Work out the finished part from the listing and answer in its coordinate system (mm). Face numbers are marked on the shaded views. A direction names the side the tool comes from. Round coordinates to 2 decimals unless told otherwise and drop trailing zeros. Order: outer loops, then holes, each group sorted by start corner. A loop starts at its lowest first (then second) coordinate and runs counter-clockwise, first axis right, second up. Notation, with made-up numbers: M 6,59.25 L 32,59.25 A28 ccw 32,89.25 Z; hole C -30.5,-22 d8. An arc over 180 degrees is marked long. Return JSON: item names as keys, results as strings.
from build123d import *

# Parameters (mm, degrees)
F0_W        = 46
F0_H        = 72
F1_DEPTH    = 96
F2_W        = 42
F2_H        = 68
F3_DEPTH    = 92
F4_R        = 4
F5_DEPTH    = 3.2
F6_R        = 4
F7_DEPTH    = 3.2
F8_T1_DEPTH = 97.7168298797
F9_R        = 1
F10_R       = 27.7209608442
F11_DEPTH   = 2


# Not quite as in the source:
# - a fillet or chamfer that OpenCascade refuses, or shapes differently, is made with other operations: its cross-section is extruded or revolved along the edge and cut away or added


with BuildPart() as f1:
    # F0 (on Top) → F1 (new body)
    with BuildSketch(Plane.XY):
        Rectangle(F0_W, F0_H)
    extrude(amount=F1_DEPTH)

    # F2 (on face) → F3 (cut)
    with BuildSketch(Plane.XY.offset(96)):
        Rectangle(F2_W, F2_H)
    extrude(amount=-F3_DEPTH, mode=Mode.SUBTRACT)

    # F4 (on face) → F5 (join)
    with BuildSketch(Plane.XZ.offset(36)):
        with Locations((13, 82)):
            Circle(F4_R)
    extrude(amount=F5_DEPTH)

    # F6 (on face) → F7 (join)
    with BuildSketch(Plane(origin=(0, 36, 0), x_dir=(-1, 0, 0), z_dir=(0, 1, 0))):
        with Locations((-13, 82)):
            Circle(F6_R)
    extrude(amount=F7_DEPTH)

    # F8: chamfer of 5 on 1 edges, made by hand

    # F8_s2 → F8_t1 (cut)
    with BuildSketch(Plane.XZ.offset(-48.8584149398)):
        Polygon((-18, 96), (-23, 91), (-23, 96), align=None)
    extrude(amount=F8_T1_DEPTH, mode=Mode.SUBTRACT)

    # F9
    f9_edges = [f1.edges().sort_by_distance(p)[0] for p in [
        (-23, -36, 45.5),
        (23, -36, 48),
        (23, 36, 48),
        (-23, 36, 45.5),
        (23, 0, 0),
        (-23, 0, 0),
        (0, 36, 0),
        (0, -36, 0),
    ]]
    fillet(f9_edges, radius=F9_R)

    # F10 (on face) → F11 (join)
    with BuildSketch(Plane(origin=(-23, 0, 0), x_dir=(0, -1, 0), z_dir=(-1, 0, 0))):
        with Locations((0, 40.8182404935)):
            Circle(F10_R)
        with BuildLine():
            add(Edge.make_bspline(
                [(-17.8310812866, 24.7516158604), (-18.0416931886, 24.731624497), (-18.6386807496, 24.6684959969), (-19.2717295968, 24.3841029538), (-19.5649090195, 21.6870798509), (-16.5966593688, 21.0684697904), (-15.2211504824, 21.4407750456), (-14.5426337104, 21.7238514822)],
                knots=[0.4132110552, 0.4132110552, 0.4132110552, 0.4132110552, 0.4283251344, 0.4603190645, 0.510541782, 0.5666924956, 0.615415561, 0.615415561, 0.615415561, 0.615415561], degree=3))
            ThreePointArc((-17.8310812866, 24.7516158604), (-8.6054277875, 63.2242776163), (24.0017475812, 40.8182404935))
            ThreePointArc((24.0017475812, 40.8182404935), (22.6894322226, 32.9904980114), (18.8959899976, 26.0187320907))
            add(Edge.make_bspline(
                [(13.5544067846, 21.0101122713), (15.1773683066, 20.8286148298), (18.6415516168, 20.5611168513), (20.2513827461, 23.1969599021), (20.017563928, 26.727985113), (19.3356446095, 26.1886613097), (18.9151411243, 26.0259448267), (18.8959899976, 26.0187320907)],
                knots=[0.4868760993, 0.4868760993, 0.4868760993, 0.4868760993, 0.6035189288, 0.7106541171, 0.8124300784, 0.8685997483, 0.87123087, 0.87123087, 0.87123087, 0.87123087], degree=3))
            ThreePointArc((13.5544067846, 21.0101122713), (-0.6095113038, 16.8242332642), (-14.5426337104, 21.7238514822))
        make_face(mode=Mode.SUBTRACT)
        with BuildLine():
            add(Edge.make_bspline(
                [(-13.1672387943, 47.9557514191), (-13.6789435568, 47.7302779724), (-13.8554780387, 46.5012200329), (-11.906507855, 43.7928351191), (-10.8613262187, 42.8100774548), (-6.4416701192, 46.0388131445), (-5.8697363247, 48.1862573802), (-6.5496625571, 49.5720681387), (-8.0107671732, 47.5720952119), (-12.18493142, 48.3885873933), (-13.1672387943, 47.9557514191)],
                knots=[0, 0, 0, 0, 0.0951179589, 0.2427295185, 0.3289680533, 0.5102542132, 0.6320447089, 0.7083203168, 0.817404333, 1, 1, 1, 1], degree=3))
        make_face()
        with BuildLine():
            add(Edge.make_bspline(
                [(-1.5056377742, 51.0721281171), (-1.2655745051, 51.376089636), (-0.785072868, 51.9844876136), (0.4890633383, 51.9466317035), (1.1904519521, 51.3741917059), (1.5605587978, 51.0721281171)],
                knots=[0, 0, 0, 0, 0.3204609859, 0.6414226921, 1, 1, 1, 1], degree=3))
            Line((-1.5056377742, 51.0721281171), (-1.5056377742, 40.8182404935))
            Line((-1.5056377742, 40.8182404935), (-13.8206910342, 40.8182404935))
            add(Edge.make_bspline(
                [(-13.8206910342, 40.8182404935), (-14.3163583008, 40.7406958322), (-15.3248298347, 40.5829255117), (-16.0298313022, 38.9853309187), (-15.2661185632, 37.3287424191), (-14.2935212413, 37.5798078265), (-13.8206910342, 37.7018637955)],
                knots=[0, 0, 0, 0, 0.2499158182, 0.5084721255, 0.7610427034, 1, 1, 1, 1], degree=3))
            Line((-13.8206910342, 37.7018637955), (-5.8284727857, 37.7018637955))
            add(Edge.make_bspline(
                [(-5.8284727857, 37.7018637955), (-5.6616792118, 37.7493233921), (-5.1463725609, 37.8959492194), (-5.9050859697, 35.7190459632), (-6.7314491211, 33.7727840823), (-8.8298986523, 30.6803066265), (-10.7443809665, 28.4421062956), (-13.4166866054, 26.493634755), (-15.5645127805, 24.9310548857), (-17.2805677978, 24.8038708143), (-17.8310812866, 24.7516158604)],
                knots=[0, 0, 0, 0, 0.0221816863, 0.0685300411, 0.1230509283, 0.1896466414, 0.2504984271, 0.3136356503, 0.3737047196, 0.4132110552, 0.4132110552, 0.4132110552, 0.4132110552], degree=3))
            ThreePointArc((-17.8310812866, 24.7516158604), (-16.2574965773, 23.1610127385), (-14.5426337104, 21.7238514822))
            add(Edge.make_bspline(
                [(-14.5426337104, 21.7238514822), (-14.4700608663, 21.7541287914), (-13.4868489797, 22.1787471182), (-11.2173445731, 23.4933801542), (-7.8402676501, 26.6128816263), (-5.3447073755, 29.9791410107), (-2.6936822721, 35.9836558885), (-2.3564969432, 37.7686367648), (-1.6866975363, 38.0047224883), (-1.4051069738, 38.1039753556)],
                knots=[0.615415561, 0.615415561, 0.615415561, 0.615415561, 0.620626886, 0.6855816442, 0.7596479515, 0.8338925842, 0.9230870978, 0.9676650246, 1, 1, 1, 1], degree=3))
            Line((-1.4051069738, 38.1039753556), (1.3092315057, 38.1039753556))
            Line((1.3092315057, 38.1039753556), (1.3092315057, 23.5273707658))
            add(Edge.make_bspline(
                [(1.3092315057, 23.5273707658), (1.3901833114, 23.1062891887), (1.5582802327, 22.2319107086), (3.1836032161, 22.2640424108), (4.3821273184, 21.9811997778), (8.5768144522, 21.4369863905), (10.9865964285, 21.3213558963), (13.0868251542, 21.0624024017), (13.5544067846, 21.0101122713)],
                knots=[0, 0, 0, 0, 0.0661108801, 0.1372796485, 0.2082189036, 0.3308717094, 0.453270839, 0.4868760993, 0.4868760993, 0.4868760993, 0.4868760993], degree=3))
            ThreePointArc((13.5544067846, 21.0101122713), (16.4173271562, 23.3095210658), (18.8959899976, 26.0187320907))
            add(Edge.make_bspline(
                [(18.8959899976, 26.0187320907), (17.958719042, 25.6657352116), (16.2187585332, 25.4761750532), (14.4787980244, 25.2866148949)],
                knots=[0.87123087, 0.87123087, 0.87123087, 0.87123087, 1, 1, 1, 1], degree=3))
            Line((14.4787980244, 25.2866148949), (4.274897743, 25.2866148949))
            Line((4.274897743, 25.2866148949), (4.274897743, 38.1039753556))
            Line((4.274897743, 38.1039753556), (14.4787980244, 38.1039753556))
            add(Edge.make_bspline(
                [(14.4787980244, 40.8182404935), (15.0214152926, 40.622477907), (15.9634432149, 40.2826180585), (15.9221942597, 39.1563781008), (15.0189015911, 38.4977733041), (14.4787980244, 38.1039753556)],
                knots=[0, 0, 0, 0, 0.3532671261, 0.6133006012, 1, 1, 1, 1], degree=3))
            Line((14.4787980244, 40.8182404935), (1.5605587978, 40.8182404935))
            Line((1.5605587978, 40.8182404935), (1.5605587978, 51.0721281171))
        make_face()
        with BuildLine():
            add(Edge.make_bspline(
                [(7.2405622341, 48.9107705653), (8.1951903629, 48.5928249221), (11.5971201687, 47.54062061), (13.8463110022, 46.6584207463), (12.1718507315, 44.887582687), (9.6429349022, 43.7513572457), (7.7599373396, 45.9568749284), (7.1288066509, 47.6332666706), (5.7942155786, 48.3483342452), (6.4651933332, 49.1853042153), (6.8443509441, 49.0427315348), (7.2405622341, 48.9107705653)],
                knots=[0, 0, 0, 0, 0.1778305446, 0.288661815, 0.3983430252, 0.5286875411, 0.6581067636, 0.7710159609, 0.8598240036, 0.9261927579, 1, 1, 1, 1], degree=3))
        make_face()
        with BuildLine():
            ThreePointArc((-14.5426337104, 21.7238514822), (-16.2574965773, 23.1610127385), (-17.8310812866, 24.7516158604))
            add(Edge.make_bspline(
                [(-17.8310812866, 24.7516158604), (-18.0416931886, 24.731624497), (-18.6386807496, 24.6684959969), (-19.2717295968, 24.3841029538), (-19.5649090195, 21.6870798509), (-16.5966593688, 21.0684697904), (-15.2211504824, 21.4407750456), (-14.5426337104, 21.7238514822)],
                knots=[0.4132110552, 0.4132110552, 0.4132110552, 0.4132110552, 0.4283251344, 0.4603190645, 0.510541782, 0.5666924956, 0.615415561, 0.615415561, 0.615415561, 0.615415561], degree=3))
        make_face()
        with BuildLine():
            ThreePointArc((18.8959899976, 26.0187320907), (16.4173271562, 23.3095210658), (13.5544067846, 21.0101122713))
            add(Edge.make_bspline(
                [(13.5544067846, 21.0101122713), (15.1773683066, 20.8286148298), (18.6415516168, 20.5611168513), (20.2513827461, 23.1969599021), (20.017563928, 26.727985113), (19.3356446095, 26.1886613097), (18.9151411243, 26.0259448267), (18.8959899976, 26.0187320907)],
                knots=[0.4868760993, 0.4868760993, 0.4868760993, 0.4868760993, 0.6035189288, 0.7106541171, 0.8124300784, 0.8685997483, 0.87123087, 0.87123087, 0.87123087, 0.87123087], degree=3))
        make_face()
    extrude(amount=F11_DEPTH)


solid = f1.part
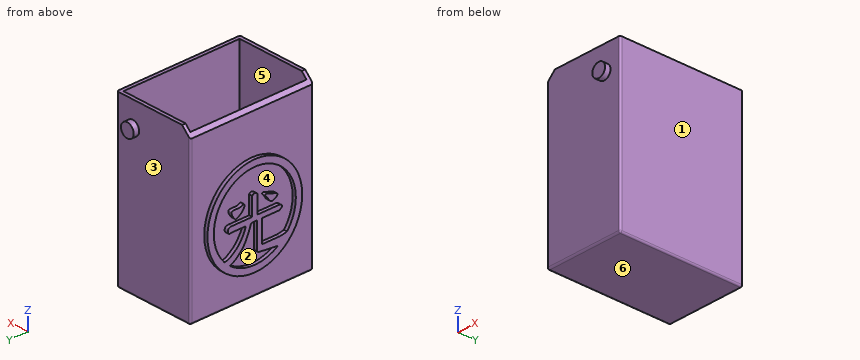
Item 1: Which of the six approach directions +Z, -Z, +X, -X, +Y, -Y give full straight-line access (tool end or side, diameter ignored) to the marked faces 4, 5 and 6?
Output:
{"face 4": "-X", "face 5": "+Z", "face 6": "-Z, +X, -X, +Y, -Y"}
Item 2: Each of these flat-tipped pins is pushed along its axis until it touches: pin 1 (0.6 mm diameter, centred on x = -24, z = 48, fed in from +Y); pin 2 (4 mm diameter, centred on y = 28, z = 54.5, fed in from -X); pin 3 (21 mm diameter, centred on x = 2, y = -6, fed in from +Z). Where does it stop, or does it pass through?
Output:
{"pin 1": "stops at y = 26.85", "pin 2": "stops at x = -23", "pin 3": "stops at z = 4"}
Item 3: Find section A-A (z = 82). Determine the outline of the cut face in (x, y), plus the area to 3 significant figures.
Output:
{"outline": "M -23,-35 A1 ccw -22,-36 L 9,-36 L 9,-39.2 L 17,-39.2 L 17,-36 L 22,-36 A1 ccw 23,-35 L 23,35 A1 ccw 22,36 L 17,36 L 17,39.2 L 9,39.2 L 9,36 L -22,36 A1 ccw -23,35 Z; hole M -21,-34 L 21,-34 L 21,34 L -21,34 Z", "area": "506 mm^2"}
Item 4: The mould has two halves that part along Y. Classify the marked faces 1, 2 and 3: pulls with the +Y half, pulls with the -Y half, needs draft (parallel to the pull), parting line crosses it, or undercut.
Output:
{"face 1": "needs draft", "face 2": "undercut", "face 3": "pulls with the +Y half"}
Item 5: Find section B-B (x = 13). Determine the outline of the cut face in (y, z), plus the area to 3 significant figures.
Output:
{"outline": "M -39.2,78 L -36,78 L -36,1 A1 ccw -35,0 L 35,0 A1 ccw 36,1 L 36,78 L 39.2,78 L 39.2,86 L 36,86 L 36,96 L 34,96 L 34,4 L -34,4 L -34,96 L -36,96 L -36,86 L -39.2,86 Z", "area": "707 mm^2"}
Item 6: Find section D-D (x = -8). Determine the outline of the cut face in (y, z), plus the area to 3 significant figures.
Output:
{"outline": "M -36,1 A1 ccw -35,0 L 35,0 A1 ccw 36,1 L 36,96 L 34,96 L 34,4 L -34,4 L -34,96 L -36,96 Z", "area": "656 mm^2"}
Item 7: Consider line 1 along Z through (x, y) = (-24.3, 0); line 2 along X through (y, z) = (8, 44); line 3 along Y through (x, z) = (13.5, 81.5). Determine where each line is inside the solid, lowest interval first. Write a range as [from, to].
Output:
{"line 1": "z = [13.1, 16.82], [38.1, 51.92], [64.82, 68.54]", "line 2": "x = [-23, -21], [21, 23]", "line 3": "y = [-39.2, -34], [34, 39.2]"}
Item 8: Find section C-C (y = 26.5). Determine the outline of the cut face in (x, z), plus the area to 3 significant figures.
Output:
{"outline": "M -25,32.68 L -23,32.68 L -23,1 A1 ccw -22,0 L 22,0 A1 ccw 23,1 L 23,96 L 21,96 L 21,4 L -21,4 L -21,93 L -23,91 L -23,48.95 L -25,48.95 Z", "area": "576 mm^2"}
